Read the model definition and answer for the solid it produces. Units are mm, in the model's axes. Face numbers are marked on the shaded views. A direction names the side the tool comes from. Coordinates: 2 decimals unless noted, no trailing zeros. Write each loop counter-clockwise with the first axis right and the second up, starting at its lowest first coordinate (ties: lowest second). Pieces come first, ordered by that corner, then holes. Notation, with made-up numbers: (66, -19) - (96, -19) arc R20 ccw to (96, -12) - close; hole circle Ø5 at (-34.5, -25.5). An arc over 180 degrees is marked (long way). Use a Markdown table: item, result.
from build123d import *

# Parameters (mm, degrees)
BOSS_EXTRUDE1_DEPTH = 0.127
SKETCH5_R           = 3.81
BOSS_EXTRUDE2_DEPTH = 8.89
CUT_EXTRUDE1_DEPTH  = 4.937
CUT_EXTRUDE3_DEPTH  = 2.54


with BuildPart() as part:
    # Sketch1 → Boss-Extrude1 (new body, symmetric)
    with BuildSketch(Plane.XY):
        with BuildLine():
            Line((0, 0), (0, 9.525))
            ThreePointArc((0, 9.525), (0.92993597, 11.77006403), (3.175, 12.7))
            Line((3.175, 12.7), (23.622, 12.7))
            Line((23.622, 12.7), (24.79704807, 11.52495193))
            Line((24.79704807, 11.52495193), (24.79704807, 7.52504807))
            Line((24.79704807, 7.52504807), (23.622, 6.35))
            Line((23.622, 6.35), (23.622, -2.286))
            Line((23.622, -2.286), (16.92369646, -2.286))
            Line((16.92369646, -2.286), (14.478, 0.15969646))
            Line((14.478, 0.15969646), (14.478, 4.445))
            ThreePointArc((14.478, 4.445), (13.54806403, 6.69006403), (11.303, 7.62))
            Line((11.303, 7.62), (7.239, 7.62))
            ThreePointArc((7.239, 7.62), (4.99393597, 6.69006403), (4.064, 4.445))
            Line((4.064, 4.445), (4.064, 0))
            Line((4.064, 0), (0, 0))
        make_face()
    extrude(amount=BOSS_EXTRUDE1_DEPTH, both=True)

    # Sketch5 → Boss-Extrude2 (add)
    with BuildSketch(Plane(origin=(24.79704807, 0, 0), x_dir=(0, 0, -1), z_dir=(1, 0, 0))):
        with Locations((0, 9.49295193)):
            Circle(SKETCH5_R)
    extrude(amount=BOSS_EXTRUDE2_DEPTH)

    # Sketch6 → Cut-Extrude1 (cut, through all)
    with BuildSketch(Plane.XY.offset(0.127)):
        Polygon((4.826, 10.922), (4.826, 8.382), (9.144, 9.652), align=None)
    extrude(amount=-CUT_EXTRUDE1_DEPTH, mode=Mode.SUBTRACT)

    # Sketch8 → Cut-Extrude3 (cut)
    with BuildSketch(Plane(origin=(0, 0, -0.127), x_dir=(-1, 0, 0), z_dir=(0, 0, -1))):
        with BuildLine():
            ThreePointArc((-10.82704807, 12.7), (-9.929022457, 12.328025612), (-9.55704807, 11.43))
            Line((-9.55704807, 11.43), (-9.55704807, 10.308777788))
            ThreePointArc((-9.55704807, 10.308777788), (-9.268748673, 9.503070692), (-8.534742676, 9.06316654))
            Line((-8.534742676, 9.06316654), (-1.022305393, 7.569289375))
            ThreePointArc((-1.022305393, 7.569289375), (-0.288299396, 7.129385223), (0, 6.323678127))
            Line((0, 6.323678127), (0, 9.525))
            ThreePointArc((0, 9.525), (-0.92993597, 11.77006403), (-3.175, 12.7))
            Line((-3.175, 12.7), (-10.82704807, 12.7))
        make_face()
        Polygon((-4.826, 8.382), (-9.144, 9.652), (-4.826, 10.922), align=None, mode=Mode.SUBTRACT)
    extrude(amount=-CUT_EXTRUDE3_DEPTH, mode=Mode.SUBTRACT)


solid = part.part
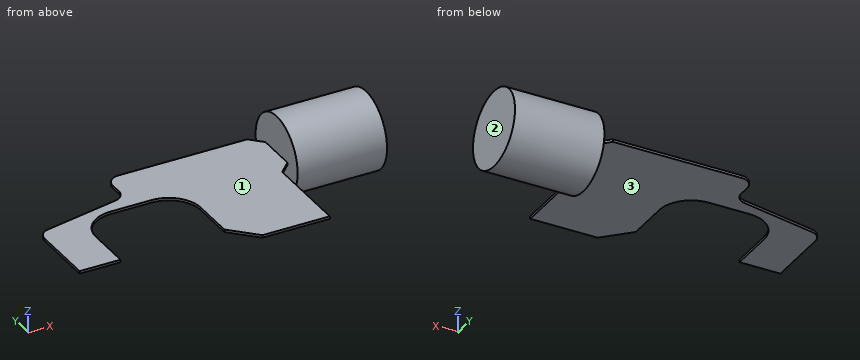
(1) For the marked faces 1, 2 and 3, determine the directions among +Z, -Z, +X, -X, +Y, -Y from which every point of the face is accessible in a straight line to the end or side of a thin tool.
Report:
| item | result |
|---|---|
| face 1 | +Z, -X, +Y, -Y |
| face 2 | +Z, -Z, +X, +Y, -Y |
| face 3 | -Z, -X, +Y, -Y |
(2) A cutting plane is placed at A-A, the plane y = 8.75. Write down the section's boundary in (x, z).
Report:
| item | result |
|---|---|
| outline | (6.96, -0.13) - (24.8, -0.13) - (24.8, -3.74) - (33.69, -3.74) - (33.69, 3.74) - (24.8, 3.74) - (24.8, 0.13) - (6.96, 0.13) - close |
(3) A cutting plane is placed at B-B, the plane z = 0.75. Write down the section's boundary in (x, y), and give its area (3 significant figures).
Report:
| item | result |
|---|---|
| outline | (24.8, 5.76) - (33.69, 5.76) - (33.69, 13.23) - (24.8, 13.23) - close |
| area | 66.4 mm² |
(4) Each of these flat-tipped pins is pushed along its axis until it touches: P1, Ø4.5, axis at x = 17, y = 3.5, coming from the +Z side; P2, Ø4, axis at y = 0, z = 1, coming from the +X side; P3, Ø1, axis at x = 27.5, z = 0.5, coming from the +Y side; P4, Ø6, axis at x = 30, y = 4, coming from the -Z side. Where does it stop, or does it pass through?
Report:
| item | result |
|---|---|
| P1 | stops at z = 0.13 |
| P2 | stops at x = 23.62 |
| P3 | stops at y = 13.3 |
| P4 | stops at z = -2.88 |
(5) Straight lines are drawn through the part: L1, parallel to Z at x = 20, y = 10; L2, parallel to X at y = 12, z = 2.5; L3, parallel to X at y = -0.5, z = 0. For each, find the intervals that lie inside material, in ascending order.
Report:
| item | result |
|---|---|
| L1 | z = -0.13 to 0.13 |
| L2 | x = 24.8 to 33.69 |
| L3 | x = 15.14 to 23.62 |
(6) A cutting plane is placed at C-C, the plane x = 12.5. Write down the section's boundary in (y, z), and give its area (3 significant figures).
Report:
| item | result |
|---|---|
| outline | (7.39, -0.13) - (12.7, -0.13) - (12.7, 0.13) - (7.39, 0.13) - close |
| area | 1.35 mm² |
